The listing builds one solid part. Answer for the finished solid, in the listing's coordinates (mm). Face numbers are marked on the shaded views. A direction names the side the tool comes from. Give positions to 0.01 mm unless a question says otherwise; leave off trailing zeros. Loops run counter-clockwise (first coordinate to the right, second up) from the corner with the lowest first, then second, coordinate; pieces in that order, holes last. Notation, with made-up numbers: (68.25, 21.25) - (90.25, 21.25) arc R18 ccw to (90.25, 56.25) - close; hole circle Ø1 at (41, 46). An arc over 180 degrees is marked (long way). Write item = value, one per line. Start each with the question number.
1) The part is cut by section C-C on y = 9.5. Write down the section's boundary in (x, z), plus the area to 3 significant figures.
2) The part is cut by section A-A on x = -0.4. Write down the section's boundary in (y, z), plus the area to 3 significant figures.
3) The part is cut by section D-D on z = -3.25. Write down the section's boundary in (x, y).
4) Which of the six approach directions +Z, -Z, +X, -X, +Y, -Y give full straight-line access (tool end or side, diameter ignored) to the marked faces 1, 2, 3, 4 and 5?
5) Flat-ended cylindrical pins translate along their axes: P1, Ø1.5, axis at x = 1.5, z = 1.5, coming from the -Y side; P2, Ø0.8, axis at x = 2, y = 7.5, coming from the -Z side; P3, Ø3, axis at y = 5, z = 2.5, coming from the -X side; P4, Ø0.8, axis at x = 1.5, y = 4, coming from the +Z side. Find the tip coordinate at first contact, or state that the pin passes through.
6) Consider probe 1 along Z at (x, y) = (-1.3, 8); probe 2 along X at (y, z) = (7.75, 6.5); probe 3 along Z at (x, y) = (0.75, 1.75). Determine where each line is inside the solid, lowest interval first.
7) The part is cut by section B-B on y = 4.5. Write down the section's boundary in (x, z), plus the area to 3 significant figures.
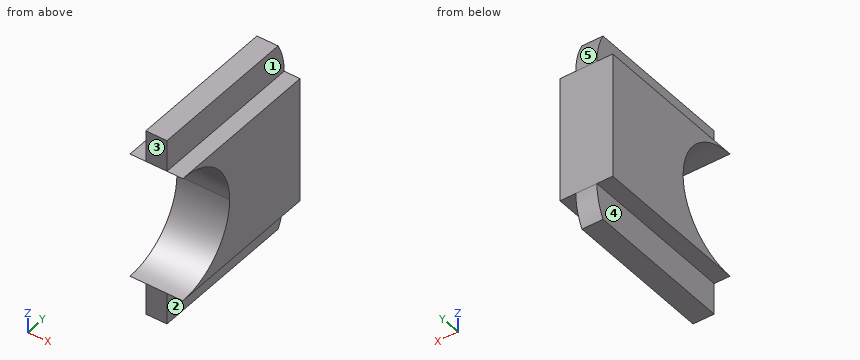
from build123d import *

# Parameters (mm, degrees)
BOSS_EXTRUDE1_DEPTH      = 2.5
BOSS_EXTRUDE1_DEPTH_BACK = 2.5
BOSS_EXTRUDE2_DEPTH      = 1
BOSS_EXTRUDE2_DEPTH_BACK = 1


with BuildPart() as part:
    # Sketch1 → Boss-Extrude1 (new, two sides: drawn at the far end of the back side and taken through both)
    with BuildSketch(Plane(origin=(0, 0, 0), x_dir=(0, 0, -1), z_dir=(1, 0, 0)).offset(-BOSS_EXTRUDE1_DEPTH_BACK)):
        with BuildLine():
            ThreePointArc((-6, 0), (-4.242640687, 4.242640687), (0, 6))
            Line((0, 6), (0, 15))
            Line((0, 15), (-6, 15))
            Line((-6, 15), (-6, 0))
        make_face()
        with BuildLine():
            Line((0, 15), (0, 6))
            ThreePointArc((0, 6), (4.242640687, 4.242640687), (6, 0))
            Line((6, 0), (6, 15))
            Line((6, 15), (0, 15))
        make_face()
    extrude(amount=BOSS_EXTRUDE1_DEPTH + BOSS_EXTRUDE1_DEPTH_BACK)

    # Sketch1_3 → Boss-Extrude2 (add, two sides: drawn at the far end of the back side and taken through both)
    with BuildSketch(Plane(origin=(0, 0, 0), x_dir=(0, 0, -1), z_dir=(1, 0, 0)).offset(-BOSS_EXTRUDE2_DEPTH_BACK)):
        with BuildLine():
            Line((-6, 0), (-6, 15))
            ThreePointArc((-6, 15), (-7.549870962, 14.801811394), (-9, 14.22))
            Line((-9, 14.22), (-9, 0))
            Line((-9, 0), (-6, 0))
        make_face()
        with BuildLine():
            ThreePointArc((9, 14.22), (7.549870962, 14.801811394), (6, 15))
            Line((6, 15), (6, 0))
            Line((6, 0), (9, 0))
            Line((9, 0), (9, 14.22))
        make_face()
    extrude(amount=BOSS_EXTRUDE2_DEPTH + BOSS_EXTRUDE2_DEPTH_BACK)


solid = part.part
Answer below:
q1.outline = (-2.5, -6) - (-1, -6) - (-1, -9) - (1, -9) - (1, -6) - (2.5, -6) - (2.5, 6) - (1, 6) - (1, 9) - (-1, 9) - (-1, 6) - (-2.5, 6) - close
q1.area = 72.0 mm2
q2.outline = (0, -9) - (14.22, -9) arc R6.16 ccw to (15, -6) - (15, 6) arc R6.16 ccw to (14.22, 9) - (0, 9) - (0, 6) arc R6 cw to (0, -6) - close
q2.area = 212 mm2
q3.outline = (-2.5, 5.04) - (2.5, 5.04) - (2.5, 15) - (-2.5, 15) - close
q4.face_1 = +Z, +X, +Y, -Y
q4.face_2 = -Z, +X, +Y, -Y
q4.face_3 = +Z, -Z, +X, -X, -Y
q4.face_4 = -Z, -X, +Y, -Y
q4.face_5 = +Z, +X, -X, +Y
q5.P1 = 5.56
q5.P2 = -6
q5.P3 = -2.5
q5.P4 = 6
q6.probe_1 = -6 to 6
q6.probe_2 = -1 to 1
q6.probe_3 = -9 to -5.74, 5.74 to 9
q7.outline = (-2.5, -6) - (-1, -6) - (-1, -9) - (1, -9) - (1, -6) - (2.5, -6) - (2.5, -3.97) - (-2.5, -3.97) - close; (-2.5, 3.97) - (2.5, 3.97) - (2.5, 6) - (1, 6) - (1, 9) - (-1, 9) - (-1, 6) - (-2.5, 6) - close
q7.area = 32.3 mm2
